Check sheet for the modelled part. Datum: model origin and axes. Units: mm. A direction names the side the tool comes from. Round coordinates to 2 decimals unless told otherwise and drop trailing zeros. Order: outer loops, then holes, each group sorted by start corner. A loop starts at its lowest first (then second) coordinate and runs counter-clockwise, first axis right, second up.
from build123d import *

# Parameters (mm, degrees)
F0_W     = 42.5828881562
F0_H     = 30.9346560389
F1_DEPTH = 56.388
F2_W     = 22.6413179189
F2_H     = 11.9935432317
F3_DEPTH = 25.4
F4_SIZE  = 5.08


with BuildPart() as f1:
    # F0 (on Front) → F1 (new body)
    with BuildSketch(Plane.XZ):
        with Locations((21.2914440781, 15.4673280194)):
            Rectangle(F0_W, F0_H)
    extrude(amount=F1_DEPTH)

    # F2 (on face) → F3 (join)
    with BuildSketch(Plane.XY.offset(30.9346560389)):
        with Locations((31.2622291967, -22.1972283841)):
            Rectangle(F2_W, F2_H)
    extrude(amount=F3_DEPTH)

    # F4
    f4_edges = [f1.edges().sort_by_distance(p)[0] for p in [
        (31.262229, -28.194, 30.934656),
        (42.582888, -42.291, 30.934656),
        (21.291444, 0, 0),
        (42.582888, 0, 15.467328),
        (42.582888, -28.194, 43.634656),
    ]]
    chamfer(f4_edges, length=F4_SIZE)


solid = f1.part
1) Sectioned sample at C-C on y = -19. Record the cut outline in (x, z).
2) Sectioned sample at D-D on x = 3. Record the cut outline in (y, z).
3) Gauge pin test, flat ends, axial feed: pin 1 (4 mm diameter, centred on x = 10, y = -19, fed in from +Z); pin 2 (5 mm diameter, centred on x = 28.5, z = 42, fed in from +Y); pin 3 (19.5 mm diameter, centred on x = 29.5, z = 45.5, fed in from -Y). Record the tip position at first contact, or that the pin passes through.
4) Set-up check for faces 1 (the face through (31, -16.2, 43)), 2 (the face through (19.942, -23, 43)), 3 (the face through (40.007, -25.69, 46.032)), 4 (the face through (29, -28.194, 46)), 5 (the face through (40.078, -2.576, 15.251)): record each of +Z, -Z, +X, -X, +Y, -Y from which the full face is reachable in a straight line by a thin tool's end or side.
5) Sectioned sample at A-A on x = 27. Record the cut outline in (y, z).
6) Scan lines: line 1 (Z direction, x = 36.5, y = -46); line 2 (Y direction, x = 24, z = 48); line 3 (X direction, y = -20.5, z = 39). Record each from-to range of solid material in increasing order.
7) Sectioned sample at B-B on z = 37. Record the cut outline in (x, y).
Values found:
1. outline: (0, 0) - (42.58, 0) - (42.58, 56.33) - (19.94, 56.33) - (19.94, 30.93) - (0, 30.93) - close
2. outline: (-56.39, 0) - (-5.08, 0) - (0, 5.08) - (0, 30.93) - (-56.39, 30.93) - close
3. pin 1: stops at z = 30.93
3. pin 2: stops at y = -16.2
3. pin 3: stops at y = -28.46
4. face 1: +Z, +X, -X, +Y
4. face 2: +Z, -X, +Y, -Y
4. face 3: +Z, +X, -Y
4. face 4: +Z, +X, -X, -Y
4. face 5: +Z, -Z, +X, +Y
5. outline: (-56.39, 0) - (-5.08, 0) - (0, 5.08) - (0, 30.93) - (-16.2, 30.93) - (-16.2, 56.33) - (-28.19, 56.33) - (-28.19, 36.01) - (-33.27, 30.93) - (-56.39, 30.93) - close
6. line 1: z = 0 to 30.93
6. line 2: y = -28.19 to -16.2
6. line 3: x = 19.94 to 42.58
7. outline: (19.94, -28.19) - (37.5, -28.19) - (42.58, -23.11) - (42.58, -16.2) - (19.94, -16.2) - close
